Geometry: final body of the model. Coordinates: model frame, mm. Give positions to 0.01 mm unless a question says otherwise; leave off trailing zeros. Order: outer loops, then holes, each group sorted by start corner. A loop starts at its lowest first (then second) coordinate and runs counter-clockwise, first axis right, second up. Notation, with made-up numbers: M -37.5,41.5 L 21.5,41.5 A15 cw 21.5,52.5 Z; hole C -20,17 d9. An arc over 180 degrees is marked long. Use CSV: the item, a comma, the result in double quotes.
```python
from build123d import *

# Parameters (mm, degrees)
SKETCH1_R            = 5
BOSS_EXTRUDE1_DEPTH  = 3
SKETCH2_R            = 1.5
CUT_EXTRUDE1_DEPTH   = 4
LPATTERN1_COUNT      = 2
LPATTERN1_PITCH      = 31
LPATTERN1_COUNT_DIR2 = 2
LPATTERN1_PITCH_DIR2 = 31
SKETCH3_R            = 2.5
CUT_EXTRUDE2_DEPTH   = 4
LPATTERN2_COUNT      = 2
LPATTERN2_PITCH      = 20
FILLET1_R            = 10
FILLET2_R            = 5


with BuildPart() as part:
    # Sketch1 → Boss-Extrude1 (new body)
    with BuildSketch(Plane(origin=(0, 0, 0), x_dir=(1, 0, 0), z_dir=(0, 1, 0))):
        Polygon((20, -20), (10, -40), (-30, -40), (-30, -20), (-20, 20), (20, 20), align=None)
        Circle(SKETCH1_R, mode=Mode.SUBTRACT)
    extrude(amount=BOSS_EXTRUDE1_DEPTH)

    # Sketch2 → Cut-Extrude1 (cut, through all)
    with BuildSketch(Plane(origin=(0, 3, 0), x_dir=(1, 0, 0), z_dir=(0, 1, 0))):
        with Locations((-15.5, 15.5)):
            Circle(SKETCH2_R)
    cut_extrude1 = extrude(amount=-CUT_EXTRUDE1_DEPTH, mode=Mode.SUBTRACT)

    # LPattern1: Cut-Extrude1 2 × 2
    with Locations(*[(i * LPATTERN1_PITCH, 0, j * LPATTERN1_PITCH_DIR2) for i in range(LPATTERN1_COUNT) for j in range(LPATTERN1_COUNT_DIR2) if (i, j) != (0, 0)]):
        add(cut_extrude1, mode=Mode.SUBTRACT)

    # Sketch3 → Cut-Extrude2 (cut, through all)
    with BuildSketch(Plane(origin=(0, 3, 0), x_dir=(1, 0, 0), z_dir=(0, 1, 0))):
        with Locations((-20, -30)):
            Circle(SKETCH3_R)
    cut_extrude2 = extrude(amount=-CUT_EXTRUDE2_DEPTH, mode=Mode.SUBTRACT)

    # LPattern2: Cut-Extrude2 ×2
    with Locations(*[(i * LPATTERN2_PITCH, 0, 0) for i in range(1, LPATTERN2_COUNT)]):
        add(cut_extrude2, mode=Mode.SUBTRACT)

    # Fillet1
    fillet1_edges = [part.edges().sort_by_distance(p)[0] for p in [
        (-30, 1.5, 40),
        (-30, 1.5, 20),
        (-20, 1.5, -20),
        (20, 1.5, 20),
        (10, 1.5, 40),
    ]]
    fillet(fillet1_edges, radius=FILLET1_R)

    # Fillet2
    fillet2_edges = [part.edges().sort_by_distance(p)[0] for p in [
        (20, 1.5, -20),
    ]]
    fillet(fillet2_edges, radius=FILLET2_R)


solid = part.part
```
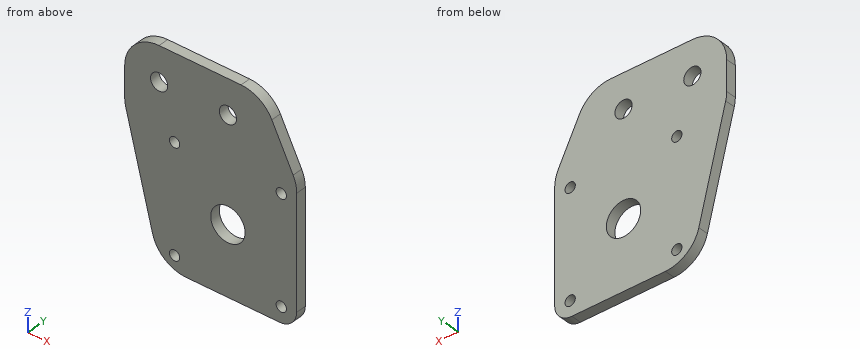
1. Section C-C, the plane z = 0. Return the cut outline in (x, y), plus the area to 3 significant figures.
Answer:
outline,"M -25,0 L -5,0 L -5,3 L -25,3 Z; M 5,0 L 20,0 L 20,3 L 5,3 Z"
area,"105 mm2"
2. Section B-B, the plane y = 0.45. Return the cut outline in (x, z), plus the area to 3 significant figures.
Answer:
outline,"M -30,21.23 A10 ccw -29.7,18.81 L -21.89,-12.43 A10 ccw -12.19,-20 L 15,-20 A5 ccw 20,-15 L 20,17.64 A10 ccw 18.94,22.11 L 12.76,34.47 A10 ccw 3.82,40 L -20,40 A10 ccw -30,30 Z; hole C -20,30 d5; hole C -15.5,-15.5 d3; hole C -15.5,15.5 d3; hole C 0,0 d10; hole C 0,30 d5; hole C 15.5,-15.5 d3; hole C 15.5,15.5 d3"
area,"2,510 mm2"
3. Section D-D, the plane z = -11. Return the cut outline in (x, y).
Answer:
outline,"M -22.25,0 L 20,0 L 20,3 L -22.25,3 Z"
4. Line query: line 1 (Z direction, x = 0, y = 2); line 2 (X direction, y = 1, z = 30); line 3 (X direction, y = 1.7, z = 15.5) (3 decimals). Output: solid intervals per line, ascending.
Answer:
line 1,"-20 to -5, 5 to 27.5, 32.5 to 40"
line 2,"-30 to -22.5, -17.5 to -2.5, 2.5 to 15"
line 3,"-28.875 to -17, -14 to 14, 17 to 20"
5. Section A-A, the plane x = 0. Return the cut outline in (y, z), plus the area to 3 significant figures.
Answer:
outline,"M 0,-20 L 3,-20 L 3,-5 L 0,-5 Z; M 0,5 L 3,5 L 3,27.5 L 0,27.5 Z; M 0,32.5 L 3,32.5 L 3,40 L 0,40 Z"
area,"135 mm2"
